from build123d import *

# Parameters (mm, degrees)
BOSS_EXTRUDE1_DEPTH   = 17.78
BOSS_EXTRUDE1_2_DEPTH = 17.78
BOSS_EXTRUDE1_3_DEPTH = 17.78
BOSS_EXTRUDE1_4_DEPTH = 17.78
SKETCH2_W             = 13.04
SKETCH2_H             = 12.04
BOSS_EXTRUDE2_DEPTH   = 17.78
SKETCH3_W             = 12.7
SKETCH3_H             = 76.2
SKETCH3_R             = 3.429
BOSS_EXTRUDE3_DEPTH   = 3.175
SKETCH4_OUTSIDE_W     = 32.334
SKETCH4_OUTSIDE_H     = 95.494
SKETCH4_OUTSIDE_W_2   = 12.7
SKETCH4_OUTSIDE_H_2   = 76.2
CUT_EXTRUDE2_DEPTH    = 55.722213268


with BuildPart() as part:
    # Sketch1 → Boss-Extrude1 (new body)
    with BuildSketch(Plane(origin=(0, 0, 0), x_dir=(1, 0, 0), z_dir=(0, 1, 0))):
        Polygon((-5.25, 4.75), (-5.25, 2.718), (-6.52, 2.718), (-6.52, 6.02), (-3.218, 6.02), (-3.218, 4.75), align=None)
    extrude(amount=BOSS_EXTRUDE1_DEPTH)



with BuildPart() as body_2:
    # Sketch1 → Boss-Extrude1 2 (new body)
    with BuildSketch(Plane(origin=(0, 0, 0), x_dir=(1, 0, 0), z_dir=(0, 1, 0))):
        Polygon((6.52, 2.718), (6.52, 6.02), (3.218, 6.02), (3.218, 4.75), (5.25, 4.75), (5.25, 2.718), align=None)
    extrude(amount=BOSS_EXTRUDE1_2_DEPTH)


with BuildPart() as body_3:
    # Sketch1 → Boss-Extrude1 3 (new body)
    with BuildSketch(Plane(origin=(0, 0, 0), x_dir=(1, 0, 0), z_dir=(0, 1, 0))):
        Polygon((5.25, -2.718), (6.52, -2.718), (6.52, -6.02), (3.218, -6.02), (3.218, -4.75), (5.25, -4.75), align=None)
    extrude(amount=BOSS_EXTRUDE1_3_DEPTH)


with BuildPart() as body_4:
    # Sketch1 → Boss-Extrude1 4 (new body)
    with BuildSketch(Plane(origin=(0, 0, 0), x_dir=(1, 0, 0), z_dir=(0, 1, 0))):
        Polygon((-5.25, -2.718), (-6.52, -2.718), (-6.52, -6.02), (-3.218, -6.02), (-3.218, -4.75), (-5.25, -4.75), align=None)
    extrude(amount=BOSS_EXTRUDE1_4_DEPTH)


with BuildPart() as part_1:
    add(part.part)

    add(body_2.part)  # Boss-Extrude2 merges body 2

    add(body_3.part)  # Boss-Extrude2 merges body 3

    add(body_4.part)  # Boss-Extrude2 merges body 4
    # Sketch2 → Boss-Extrude2 (add)
    with BuildSketch(Plane(origin=(0, 0, 0), x_dir=(-1, 0, 0), z_dir=(0, -1, 0))):
        Rectangle(SKETCH2_W, SKETCH2_H)
    extrude(amount=BOSS_EXTRUDE2_DEPTH)

    # Sketch3 → Boss-Extrude3 (add)
    with BuildSketch(Plane(origin=(0, -17.78, 0), x_dir=(-1, 0, 0), z_dir=(0, -1, 0))):
        Rectangle(SKETCH3_W, SKETCH3_H)
        with Locations(Location((0, 31.75, 0), (0, 0, 90))):
            Circle(SKETCH3_R, mode=Mode.SUBTRACT)
        with Locations(Location((0, -31.75, 0), (0, 0, 270))):
            Circle(SKETCH3_R, mode=Mode.SUBTRACT)
    extrude(amount=BOSS_EXTRUDE3_DEPTH)

    # Sketch4 outside → Cut-Extrude2 (cut, through all)
    with BuildSketch(Plane.XZ.offset(20.955)):
        Rectangle(SKETCH4_OUTSIDE_W, SKETCH4_OUTSIDE_H)
        Rectangle(SKETCH4_OUTSIDE_W_2, SKETCH4_OUTSIDE_H_2, mode=Mode.SUBTRACT)
    extrude(amount=-CUT_EXTRUDE2_DEPTH, mode=Mode.SUBTRACT)


solid = part_1.part
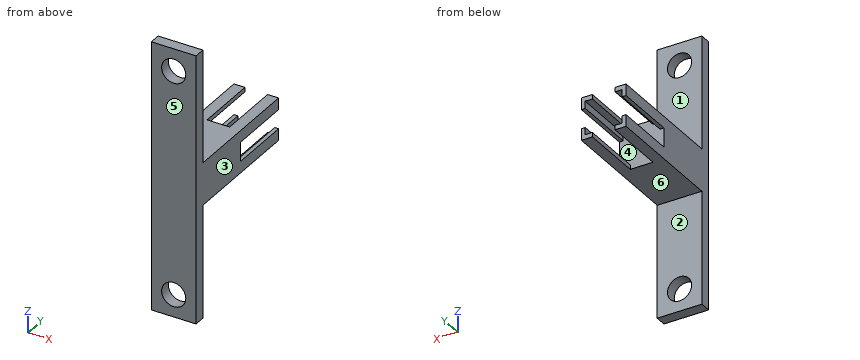
The model under review builds one solid part; all positions refer to its coordinate system, in mm. Face numbers are marked on the shaded views. A direction names the side the tool comes from. Coordinates: 2 decimals unless noted, no trailing zeros. Write each loop counter-clockwise with the first axis right and the second up, starting at its lowest first coordinate (ties: lowest second). Pieces come first, ordered by that corner, then holes. Notation, with made-up numbers: M 22.25,-1.75 L 66.25,-1.75 A16 cw 66.25,7.25 Z; hole C -34.5,36.5 d11. An arc over 180 degrees is marked long. Put each result on its own line as item: value.
1) Add section D-D on y = -14. Give the boundary of the cut face in (x, z).
Computed:
outline: M -6.35,-6.02 L 6.35,-6.02 L 6.35,6.02 L -6.35,6.02 Z
2) Draft analysis for pull direction Z (two halves, no side actions). For the marked faces 4, 5 and 6, state which applies: released by +Z, released by -Z, zero draft, split by the parting line, or undercut.
Computed:
face 4: undercut
face 5: zero draft
face 6: released by -Z
3) For the marked faces 1, 2 and 3, list the 3-axis set-ups (+Z, -Z, +X, -X, +Y, -Y) from which the entire face can be reached by the end or side of a thin tool; tool diameter is ignored.
Computed:
face 1: +Z, +X, -X, +Y
face 2: -Z, +X, -X, +Y
face 3: +Z, -Z, +X, +Y, -Y
4) Clearance check with flat-ended pins moving along their axes: pin 1 Ø2 at (x, y) = (4.5, 10) entering from -Z; pin 2 Ø0.5 at (x, y) = (-6, 9.5) entering from +Z; pin 3 Ø5.5 at (x, z) = (0, -31.75) entering from +Y; pin 4 Ø4 at (x, z) = (-3, -15) entering from +Y. State where each tip first meets the part, or that it passes through.
Computed:
pin 1: stops at z = -6.02
pin 2: stops at z = 6.02
pin 3: passes through
pin 4: stops at y = -17.78
5) Add section B-B on z = -31.75. Give the boundary of the cut face in (x, y) (3 decimals).
Computed:
outline: M -6.35,-20.955 L -3.429,-20.955 L -3.429,-17.78 L -6.35,-17.78 Z; M 3.429,-20.955 L 6.35,-20.955 L 6.35,-17.78 L 3.429,-17.78 Z
6) Wall thickness on probe 1 along Z at (x, y) = (-3.75, 6); probe 2 along X at (y, z) = (-19.9, -31.75); probe 3 along Z at (x, y) = (-0.75, -18): over which ranges is each line inside the solid? List them lowest first. Write a range as [from, to].
Computed:
probe 1: z = [-6.02, -4.75], [4.75, 6.02]
probe 2: x = [-6.35, -3.43], [3.43, 6.35]
probe 3: z = [-38.1, -35.1], [-28.4, 28.4], [35.1, 38.1]
7) Add section C-C on x = 0. Give the boundary of the cut face in (y, z) (3 decimals), then the cut area to 3 significant figures.
Computed:
outline: M -20.955,-38.1 L -17.78,-38.1 L -17.78,-35.179 L -20.955,-35.179 Z; M -20.955,-28.321 L -17.78,-28.321 L -17.78,-6.02 L 0,-6.02 L 0,6.02 L -17.78,6.02 L -17.78,28.321 L -20.955,28.321 Z; M -20.955,35.179 L -17.78,35.179 L -17.78,38.1 L -20.955,38.1 Z
area: 412 mm2
8) Add section A-A on y = 14. Give the boundary of the cut face in (x, z).
Computed:
outline: M -6.35,-6.02 L -3.22,-6.02 L -3.22,-4.75 L -5.25,-4.75 L -5.25,-2.72 L -6.35,-2.72 Z; M -6.35,2.72 L -5.25,2.72 L -5.25,4.75 L -3.22,4.75 L -3.22,6.02 L -6.35,6.02 Z; M 3.22,-6.02 L 6.35,-6.02 L 6.35,-2.72 L 5.25,-2.72 L 5.25,-4.75 L 3.22,-4.75 Z; M 3.22,4.75 L 5.25,4.75 L 5.25,2.72 L 6.35,2.72 L 6.35,6.02 L 3.22,6.02 Z
